Build history of the part. All positions in model axes, mm. Coordinates: 2 decimals unless noted, no trailing zeros. Write each loop counter-clockwise with the first axis right and the second up, starting at its lowest first coordinate (ties: lowest second). Pieces come first, ordered by that corner, then holes.
Autodesk Inventor part; units mm, degrees
ref_plane "YZ Plane" through (0, 0, 0) normal (1, 0, 0) x (0, 1, 0)
ref_plane "XZ Plane" through (0, 0, 0) normal (0, 1, 0) x (-1, 0, 0)
ref_plane "XY Plane" through (0, 0, 0) normal (0, 0, 1) x (1, 0, 0)
sketch "Sketch1" plane through (0, 0, 0) normal (0, 1, 0) x (-1, 0, 0)
  line L0 (0, 0) -> (120, 0)
  line L1 (120, 0) -> (120, -75)
  line L2 (120, -75) -> (0, -75)
  line L3 (0, -75) -> (0, 0)
  line L4 (120, 0) -> (117.5, 0)
  line L5 (117.5, 0) -> (117.5, -2.5)
  line L6 (117.5, -2.5) -> (120, -2.5)
  line L7 (120, -2.5) -> (120, 0)
  line L8 (120, -75) -> (117.5, -75)
  line L9 (117.5, -75) -> (117.5, -72.5)
  line L10 (117.5, -72.5) -> (120, -72.5)
  line L11 (120, -72.5) -> (120, -75)
  line L12 (0, -75) -> (2.5, -75)
  line L13 (2.5, -75) -> (2.5, -72.5)
  line L14 (2.5, -72.5) -> (0, -72.5)
  line L15 (0, -72.5) -> (0, -75)
  line L16 (0, 0) -> (2.5, 0)
  line L17 (2.5, 0) -> (2.5, -2.5)
  line L18 (2.5, -2.5) -> (0, -2.5)
  line L19 (0, -2.5) -> (0, 0)
  line L20 (0, 0) -> (5, 0)
  line L21 (5, 0) -> (5, -5)
  line L22 (5, -5) -> (0, -5)
  line L23 (0, -5) -> (0, 0)
  line L24 (0, -75) -> (5, -75)
  line L25 (5, -75) -> (5, -70)
  line L26 (5, -70) -> (0, -70)
  line L27 (0, -70) -> (0, -75)
  line L28 (120, 0) -> (115, 0)
  line L29 (115, 0) -> (115, -5)
  line L30 (115, -5) -> (120, -5)
  line L31 (120, -5) -> (120, 0)
  line L32 (120, -75) -> (115, -75)
  line L33 (115, -75) -> (115, -70)
  line L34 (115, -70) -> (120, -70)
  line L35 (120, -70) -> (120, -75)
  circle A0 centre (117.5, -72.5) radius 1
  circle A1 centre (117.5, -2.5) radius 1
  circle A2 centre (2.5, -2.5) radius 1
  circle A3 centre (2.5, -72.5) radius 1
  line L36 (0, 0) -> (0, -37.5)
  line L37 (0, -37.5) -> (120, -37.5)
  line L38 (60, 0) -> (60, -75)
  line L39 (0, -32.5) -> (120, -32.5)
  line L40 (120, -32.5) -> (120, -42.5)
  line L41 (120, -42.5) -> (0, -42.5)
  line L42 (0, -42.5) -> (0, -32.5)
  line L43 (0, -32.5) -> (120, -42.5) construction
  line L44 (120, -32.5) -> (0, -42.5) construction
  line L45 (55, 0) -> (65, 0)
  line L46 (65, 0) -> (65, -75)
  line L47 (65, -75) -> (55, -75)
  line L48 (55, -75) -> (55, 0)
  line L49 (55, 0) -> (65, -75) construction
  line L50 (65, 0) -> (55, -75) construction
  point P0 (60, -37.5)
  point P1 (60, -37.5)
  point P2 (55, -32.5)
  point P3 (55, -42.5)
  point P4 (65, -42.5)
  point P5 (65, -32.5)
  dimension "d0" = 120
  dimension "d1" = 75
  dimension "d2" = 2.5
  dimension "d3" = 2.5
  dimension "d4" = 2.5
  dimension "d5" = 2.5
  dimension "d6" = 2.5
  dimension "d7" = 2.5
  dimension "d8" = 2.5
  dimension "d9" = 2.5
  dimension "d10" = 5
  dimension "d11" = 5
  dimension "d12" = 5
  dimension "d13" = 5
  dimension "d14" = 5
  dimension "d15" = 5
  dimension "d16" = 5
  dimension "d17" = 5
  dimension "d18" = 2
  dimension "d19" = 2
  dimension "d20" = 2
  dimension "d21" = 2
  dimension "d22" = 10
  dimension "d23" = 10
extrude "Extrusion1" add sketch "Sketch1" along normal blind 0.25 contours L0 L17 A2 L18 L3 | L0 L21 L22 L3 L18 A2 L17 | L0 L48 L39 L3 L22 L21 | L0 L38 L39 L48 | L39 L48 L37 L3 | L0 L46 L39 L38 | L39 L38 L37 L48 | L37 L48 L41 L3 | L0 L29 L30 L1 L39 L46 | L39 L46 L37 L38 | L37 L38 L41 L48 | L41 L48 L2 L25 L26 L3 | L0 L5 A1 L6 L1 L30 L29 | L39 L1 L37 L46 | L37 L46 L41 L38 | L41 L38 L2 L48 | L26 L25 L2 L13 A3 L14 L3 | L0 L1 L6 A1 L5 | L37 L1 L41 L46 | L41 L46 L2 L38 | L14 A3 L13 L2 L3 | L41 L1 L34 L33 L2 L46 | L1 L10 A0 L9 L2 L33 L34 | L1 L2 L9 A0 L10
extrude "Extrusion2" add sketch "Sketch1" against normal blind 1 contours L0 L17 A2 L18 L3 | L0 L21 L22 L3 L18 A2 L17 | L0 L38 L39 L48 | L39 L48 L37 L3 | L0 L46 L39 L38 | L39 L38 L37 L48 | L37 L48 L41 L3 | L39 L46 L37 L38 | L37 L38 L41 L48 | L0 L5 A1 L6 L1 L30 L29 | L39 L1 L37 L46 | L37 L46 L41 L38 | L41 L38 L2 L48 | L26 L25 L2 L13 A3 L14 L3 | L0 L1 L6 A1 L5 | L37 L1 L41 L46 | L41 L46 L2 L38 | L14 A3 L13 L2 L3 | L1 L10 A0 L9 L2 L33 L34 | L1 L2 L9 A0 L10
properties part number "yellow_plate_cover"
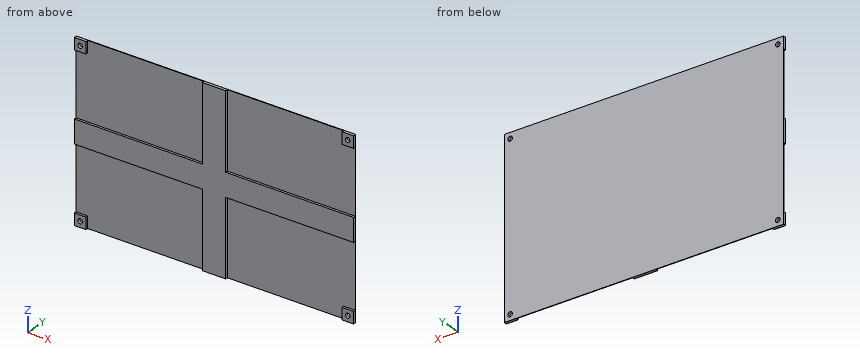
1. Flat gauge pins, fed straight in: pin 1 (5 mm diameter, centred on x = -32, z = -63.5, fed in from -Y); pin 2 (0.5 mm diameter, centred on x = -91.5, y = -0.5, fed in from -Z). Where does each tip first touch, or does it go through?
Computed values:
pin 1: stops at y = 0
pin 2: stops at z = -42.5
2. Saw through at B-B on x = -72. List the corners of the cut face in (y, z).
Computed values:
outline: (-1, -42.5) - (0, -42.5) - (0, -75) - (0.25, -75) - (0.25, 0) - (0, 0) - (0, -32.5) - (-1, -32.5) - close
3. Saw through at A-A on y = -0.35. State how many separate pieces and enclosed holes the cut face has, plus the area to 3 significant figures.
Computed values:
separate pieces: 5
enclosed holes: 4
area: 1,940 mm2
4. Probe line 1 along X through (y, z) = (-0.1, -72.5); line 2 along Z through (x, y) = (-2.5, 0.05); line 3 along Z through (x, y) = (-117.5, -0.65). List the from-to ranges inside material, lowest first.
Computed values:
line 1: x = -120 to -118.5, -116.5 to -115, -65 to -55, -5 to -3.5, -1.5 to 0
line 2: z = -75 to -73.5, -71.5 to -3.5, -1.5 to 0
line 3: z = -75 to -73.5, -71.5 to -70, -42.5 to -32.5, -5 to -3.5, -1.5 to 0
5. Saw through at C-C on z = -12.5. List the corners of the cut face in (x, y).
Computed values:
outline: (-120, 0) - (-65, 0) - (-65, -1) - (-55, -1) - (-55, 0) - (0, 0) - (0, 0.25) - (-120, 0.25) - close
